Part model, mm, in its own coordinate system. A direction names the side the tool comes from. Round coordinates to 2 decimals unless told otherwise and drop trailing zeros. Loops run counter-clockwise (first coordinate to the right, second up) from the corner with the lowest first, then second, coordinate; pieces in that order, holes last.
(1) Cut at B-B on x = 46. List the corners of the cut face in (y, z).
(2) Mould opens along Y. For faces 1 (the face through (-1, 0, 0)), 2 (the face through (56, 97.7, 22)), 3 (the face through (54.1, 96.7, -20.8)), 4 (the face through (-74.5, 44, 0)) say: +Y half, -Y half, draft (parallel to the pull), parting line (faces both ways), or undercut.
(3) Flat gauge pins, fed straight in: pin 1 (6.5 mm diameter, centred on x = 66.5, z = -8, fed in from +Y); pin 2 (1.1 mm diameter, centred on y = 97.5, z = 21, fed in from -X); pin 3 (0.5 mm diameter, centred on x = 54, y = 97.5, fed in from -Z). Where does each tip first touch, or does it go through?
(4) Tool access for faces 5 (the face through (-9, 92, 31.35)), 6 (the face through (-73.85, 92, 0)), 7 (the face through (-11, 92, -31.35)), 8 (the face through (-1, 46, 32)), 9 (the face through (54.1, 96.7, 20.8)): list every direction of +Z, -Z, +X, -X, +Y, -Y with a clear straight run to the whole face (end or side of a thin tool).
(5) Probe probe 1 along X at (y, z) = (93.5, -9.5); probe 2 along X at (y, z) = (93, 9); probe 3 along Y at (x, z) = (-50, -9.5). List the from-to ranges inside material, lowest first.
(6) Cut at A-A on y = 91. List the corners of the cut face in (x, z), then the cut area to 3 significant figures.
from build123d import *

# Parameters (mm, degrees)
SKETCH1_W            = 149
SKETCH1_H            = 64
BOSS_EXTRUDE1_DEPTH  = 93.6
SKETCH2_W            = 1.5
SKETCH2_H            = 20
CUT_EXTRUDE1_DEPTH   = 4.2
SKETCH2_3_W          = 15
SKETCH2_3_H          = 14
CUT_EXTRUDE2_DEPTH   = 0.1
SKETCH2_4_R          = 3
SKETCH2_4_W          = 5
SKETCH2_4_H          = 1
CUT_EXTRUDE3_DEPTH   = 0.2
SKETCH3_W            = 1
SKETCH3_H            = 6.6
BOSS_EXTRUDE2_DEPTH  = 4.2
SKETCH4_W            = 6.6
SKETCH4_H            = 1
BOSS_EXTRUDE3_DEPTH  = 9.1
CUT_EXTRUDE4_REACH   = 128.963
SKETCH5_W            = 3
SKETCH5_H            = 1
FILLET1_START        = 93.5
FILLET1_DEPTH        = 5.5
FILLET1_START_2      = 96.7
FILLET1_2_DEPTH      = 1
FILLET2_R            = 1.5
FILLET2_OF_MIRROR1_R = 1.5


with BuildPart() as part:
    # Sketch1 → Boss-Extrude1 (new body)
    with BuildSketch(Plane(origin=(0, 0, 0), x_dir=(1, 0, 0), z_dir=(0, 1, 0))):
        Rectangle(SKETCH1_W, SKETCH1_H)
    extrude(amount=BOSS_EXTRUDE1_DEPTH)

    # Sketch2 → Cut-Extrude1 (cut)
    with BuildSketch(Plane(origin=(0, 93.6, 0), x_dir=(1, 0, 0), z_dir=(0, 1, 0))):
        with Locations((73.75, 0)):
            Rectangle(SKETCH2_W, SKETCH2_H)
        Polygon((74.5, 10), (74.5, 11.5), (73, 10), align=None)
        Polygon((73, -10), (74.5, -11.5), (74.5, -10), align=None)
        Polygon((54.15, -32), (53.5, -31.35), (-73.85, -31.35), (-73.85, 31.35), (53.5, 31.35), (54.15, 32), (-74.5, 32), (-74.5, -32), align=None)
    extrude(amount=-CUT_EXTRUDE1_DEPTH, mode=Mode.SUBTRACT)

    # Sketch2<3> → Cut-Extrude2 (cut)
    with BuildSketch(Plane(origin=(0, 93.6, 0), x_dir=(1, 0, 0), z_dir=(0, 1, 0))):
        with Locations((63.5, 21.5)):
            Rectangle(SKETCH2_3_W, SKETCH2_3_H)
        with Locations((63.5, -21.5)):
            Rectangle(SKETCH2_3_W, SKETCH2_3_H)
    extrude(amount=-CUT_EXTRUDE2_DEPTH, mode=Mode.SUBTRACT)

    # Sketch2<4> → Cut-Extrude3 (cut)
    # profile 1 of 2: a face of its own
    with BuildSketch(Plane(origin=(0, 93.6, 0), x_dir=(1, 0, 0), z_dir=(0, 1, 0))):
        with Locations(Location((65.5, 9.5, 0), (0, 0, 270))):
            Circle(SKETCH2_4_R)
        with Locations((65.5, 9.5)):
            Rectangle(SKETCH2_4_W, SKETCH2_4_H, mode=Mode.SUBTRACT)
    # profile 2 of 2: a face of its own
    with BuildSketch(Plane(origin=(0, 93.6, 0), x_dir=(1, 0, 0), z_dir=(0, 1, 0))):
        with Locations(Location((65.5, -9.5, 0), (0, 0, 270))):
            Circle(SKETCH2_4_R)
        Polygon((68, -9), (68, -10), (66, -10), (66, -12), (65, -12), (65, -10), (63, -10), (63, -9), (65, -9), (65, -7), (66, -7), (66, -9), align=None, mode=Mode.SUBTRACT)
    extrude(amount=-CUT_EXTRUDE3_DEPTH, mode=Mode.SUBTRACT)

    # Sketch3 → Boss-Extrude2 (add)
    with BuildSketch(Plane(origin=(0, 93.5, 0), x_dir=(1, 0, 0), z_dir=(0, 1, 0))):
        with Locations((60, 21.5)):
            Rectangle(SKETCH3_W, SKETCH3_H)
    boss_extrude2 = extrude(amount=BOSS_EXTRUDE2_DEPTH)

    # Sketch4 → Boss-Extrude3 (add)
    with BuildSketch(Plane.ZY.offset(-59.5)):
        with Locations((-21.5, 97.2)):
            Rectangle(SKETCH4_W, SKETCH4_H)
    boss_extrude3 = extrude(amount=BOSS_EXTRUDE3_DEPTH)

    # Sketch5 → Cut-Extrude4 (cut, up to next)
    with BuildSketch(Plane(origin=(0, 97.7, 0), x_dir=(1, 0, 0), z_dir=(0, 1, 0)), mode=Mode.PRIVATE) as cut_extrude4_sk1:
        Polygon((57.5, 23.8), (57.5, 24.8), (49.983191487, 24.8), (49.983191487, 22.8), (50.983191487, 23.8), align=None)
    cut_extrude4_tool1 = extrude(cut_extrude4_sk1.sketch, amount=-CUT_EXTRUDE4_REACH, mode=Mode.PRIVATE) & part.part
    # Sketch5 → Cut-Extrude4 (cut, up to next)
    with BuildSketch(Plane(origin=(0, 97.7, 0), x_dir=(1, 0, 0), z_dir=(0, 1, 0)), mode=Mode.PRIVATE) as cut_extrude4_sk2:
        Polygon((57.5, 18.2), (57.5, 19.2), (50.983191487, 19.2), (49.983191487, 20.2), (49.983191487, 18.2), align=None)
    cut_extrude4_tool2 = extrude(cut_extrude4_sk2.sketch, amount=-CUT_EXTRUDE4_REACH, mode=Mode.PRIVATE) & part.part
    # Sketch5 → Cut-Extrude4 (cut, up to next)
    with BuildSketch(Plane(origin=(0, 97.7, 0), x_dir=(1, 0, 0), z_dir=(0, 1, 0)), mode=Mode.PRIVATE) as cut_extrude4_sk3:
        with Locations((53.483191487, 21.5)):
            Rectangle(SKETCH5_W, SKETCH5_H)
    cut_extrude4_tool3 = extrude(cut_extrude4_sk3.sketch, amount=-CUT_EXTRUDE4_REACH, mode=Mode.PRIVATE) & part.part
    cut_extrude4_1 = cut_extrude4_tool1.solids().sort_by_distance((53.527978, 97.7, -24.248026))[0]
    add(cut_extrude4_1, mode=Mode.SUBTRACT)
    cut_extrude4_2 = cut_extrude4_tool2.solids().sort_by_distance((53.527978, 97.7, -18.751974))[0]
    add(cut_extrude4_2, mode=Mode.SUBTRACT)
    cut_extrude4_3 = cut_extrude4_tool3.solids().sort_by_distance((53.483191, 97.7, -21.5))[0]
    add(cut_extrude4_3, mode=Mode.SUBTRACT)
    cut_extrude4 = cut_extrude4_1 + cut_extrude4_2 + cut_extrude4_3  # Cut-Extrude4 as one shape, for the pattern or mirror that repeats it

    # Fillet1: read off the stored shape, not the designer's step
    # Fillet1 outline → Fillet1 (cut)
    with BuildSketch(Plane(origin=(0, 0, 0), x_dir=(1, 0, 0), z_dir=(0, 1, 0)).offset(FILLET1_START)):
        with BuildLine():
            ThreePointArc((58, 18.2), (57.646446609, 18.346446609), (57.5, 18.7))
            Line((57.5, 18.7), (57.5, 18.2))
            Line((57.5, 18.2), (58, 18.2))
        make_face()
        with BuildLine():
            Line((57.5, 24.8), (57.5, 24.3))
            ThreePointArc((57.5, 24.3), (57.646446609, 24.653553391), (58, 24.8))
            Line((58, 24.8), (57.5, 24.8))
        make_face()
    fillet1 = extrude(amount=FILLET1_DEPTH, mode=Mode.SUBTRACT)

    # Fillet1 2 outline → Fillet1 2 (add)
    with BuildSketch(Plane(origin=(0, 0, 0), x_dir=(1, 0, 0), z_dir=(0, 1, 0)).offset(FILLET1_START_2)):
        with BuildLine():
            ThreePointArc((57, 19.2), (57.353553391, 19.053553391), (57.5, 18.7))
            Line((57.5, 18.7), (57.5, 19.2))
            Line((57.5, 19.2), (57, 19.2))
        make_face()
        with BuildLine():
            Line((57.5, 23.8), (57.5, 24.3))
            ThreePointArc((57.5, 24.3), (57.353553391, 23.946446609), (57, 23.8))
            Line((57, 23.8), (57.5, 23.8))
        make_face()
    fillet1_2 = extrude(amount=FILLET1_2_DEPTH)

    # Fillet2
    fillet2_edges = [part.edges().sort_by_distance(p)[0] for p in [
        (59.5, 96.7, -21.5),
        (60.5, 97.7, -21.5),
    ]]
    fillet(fillet2_edges, radius=FILLET2_R)

    # Mirror1: Boss-Extrude2, Boss-Extrude3, Cut-Extrude4, Fillet1, Fillet1 2 across plane
    add(boss_extrude2.mirror(Plane.XY))
    add(boss_extrude3.mirror(Plane.XY))
    add(cut_extrude4.mirror(Plane.XY), mode=Mode.SUBTRACT)
    add(fillet1.mirror(Plane.XY), mode=Mode.SUBTRACT)
    add(fillet1_2.mirror(Plane.XY))

    # Fillet2 of Mirror1
    fillet2_of_mirror1_edges = [part.edges().sort_by_distance(p)[0] for p in [
        (59.5, 96.7, 21.5),
        (60.5, 97.7, 21.5),
    ]]
    fillet(fillet2_of_mirror1_edges, radius=FILLET2_OF_MIRROR1_R)


solid = part.part
Final values:
1. outline: (0, -32) - (89.4, -32) - (89.4, -31.35) - (93.6, -31.35) - (93.6, 31.35) - (89.4, 31.35) - (89.4, 32) - (0, 32) - close
2. face 1: -Y half
2. face 2: +Y half
2. face 3: undercut
2. face 4: draft
3. pin 1: stops at y = 93.6
3. pin 2: stops at x = 50.4
3. pin 3: stops at z = -23.8
4. face 5: +Z, -X, +Y
4. face 6: +Z, -Z, -X, +Y
4. face 7: -Z, -X, +Y
4. face 8: +Z, +X, -X, +Y, -Y
4. face 9: +Z, -Z, -X
5. probe 1: x = -73.85 to 62.5, 63 to 68, 68.5 to 73
5. probe 2: x = -73.85 to 73
5. probe 3: y = 0 to 93.6
6. outline: (-73.85, -31.35) - (53.5, -31.35) - (54.15, -32) - (74.5, -32) - (74.5, -11.5) - (73, -10) - (73, 10) - (74.5, 11.5) - (74.5, 32) - (54.15, 32) - (53.5, 31.35) - (-73.85, 31.35) - close
6. area: 9,300 mm2
